Autodesk Inventor part; units mm, degrees
ref_plane "YZ Plane" through (0, 0, 0) normal (1, 0, 0) x (0, 1, 0)
ref_plane "XZ Plane" through (0, 0, 0) normal (0, 1, 0) x (-1, 0, 0)
ref_plane "XY Plane" through (0, 0, 0) normal (0, 0, 1) x (1, 0, 0)
sketch "Sketch1" plane through (0, 0, 0) normal (0, 0, 1) x (1, 0, 0)
  line L0 (0, 0) -> (-400, 0)
  line L1 (-400, 0) -> (-400, 30)
  line L2 (-400, 30) -> (0, 30)
  line L3 (0, 30) -> (0, 0)
  circle A0 centre (-15, 15) radius 5
  circle A1 centre (-85, 15) radius 5
  circle A2 centre (-315, 15) radius 5
  circle A3 centre (-385, 15) radius 5
  dimension "d0" = 400
  dimension "d1" = 30
  dimension "d2" = 10
  dimension "d3" = 10
  dimension "d4" = 10
  dimension "d5" = 10
  dimension "d6" = 15
  dimension "d7" = 15
  dimension "d8" = 15
  dimension "d9" = 70
  dimension "d10" = 15
  dimension "d11" = 15
  dimension "d12" = 70
  dimension "d13" = 15
sketch "Sketch2" plane through (0, 0, 0) normal (0, 0, 1) x (1, 0, 0)
  point P0 (0, 0)
extrude "Extrusion1" add sketch "Sketch1" along normal blind 20
properties part number "seatButtSidePlate" material "Wood (Birch)"
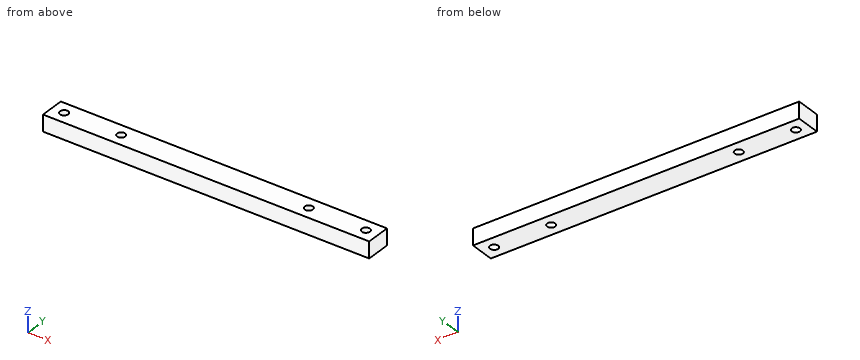
Here's how the part is built. I have some questions about the finished solid (model axes, mm). Give positions to 0.01 mm unless a question says otherwise; leave off trailing zeros. Loops run counter-clockwise (first coordinate to the right, second up) from the corner with the lowest first, then second, coordinate; pieces in that order, holes last. Notation, with made-up numbers: (23.5, 49) -> (44.5, 49) arc R20 ccw to (44.5, 59) -> close; hole circle Ø8 at (34, -18.5). An arc over 180 degrees is marked (long way). Answer as a JSON object with one key per item and string values. Group by question number.
Item 1: Imagine slicing it at C-C on z = 12.5. Write out the boundary of the cut face in (x, y), then the cut area to 3 significant figures.
Item 2: Will these pins go through, and if not, where does the flat tip stop? pin 1 (9 mm diameter, centred on x = -385, y = 15, fed in from +Z); pin 2 (12 mm diameter, centred on y = 16.5, z = 5.5, fed in from +X).
Item 3: I need wall thicknesses on L1, parallel to X at y = 14.25, z = 4; L2, parallel to Y at x = -15, z = 10; L3, parallel to X at y = 18, z = 2.5. Which ranges of each line are inside material? Lowest first, please.
Item 4: Imagine slicing it at A-A on x = -85. Write out the boundary of the cut face in (y, z), then the cut area to 3 significant figures.
Item 5: Imagine slicing it at B-B on y = 15. Write out the boundary of the cut face in (x, z), then the cut area to 3 significant figures.
Answer list:
{
 "1": {"outline": "(-400, 0) -> (0, 0) -> (0, 30) -> (-400, 30) -> close; hole circle Ø10 at (-385, 15); hole circle Ø10 at (-315, 15); hole circle Ø10 at (-85, 15); hole circle Ø10 at (-15, 15)", "area": "11,700 mm2"},
 "2": {"pin 1": "passes through", "pin 2": "stops at x = 0"},
 "3": {"L1": "x = -400 to -389.94, -380.06 to -319.94, -310.06 to -89.94, -80.06 to -19.94, -10.06 to 0", "L2": "y = 0 to 10, 20 to 30", "L3": "x = -400 to -389, -381 to -319, -311 to -89, -81 to -19, -11 to 0"},
 "4": {"outline": "(0, 0) -> (10, 0) -> (10, 20) -> (0, 20) -> close; (20, 0) -> (30, 0) -> (30, 20) -> (20, 20) -> close", "area": "400 mm2"},
 "5": {"outline": "(-400, 0) -> (-390, 0) -> (-390, 20) -> (-400, 20) -> close; (-380, 0) -> (-320, 0) -> (-320, 20) -> (-380, 20) -> close; (-310, 0) -> (-90, 0) -> (-90, 20) -> (-310, 20) -> close; (-80, 0) -> (-20, 0) -> (-20, 20) -> (-80, 20) -> close; (-10, 0) -> (0, 0) -> (0, 20) -> (-10, 20) -> close", "area": "7,200 mm2"}
}
